```python
from build123d import *

# Parameters (mm, degrees)
SKETCH1_W           = 50
SKETCH1_H           = 10
BOSS_EXTRUDE1_DEPTH = 60
CHAMFER1_SIZE       = 3
CHAMFER1_SIZE2      = 8.242432258
CHAMFER2_SIZE       = 3
CHAMFER2_SIZE2      = 8.242432258


with BuildPart() as part:
    # Sketch1 → Boss-Extrude1 (new body)
    with BuildSketch(Plane(origin=(0, 0, 0), x_dir=(0, 0, -1), z_dir=(1, 0, 0))):
        Rectangle(SKETCH1_W, SKETCH1_H)
    extrude(amount=BOSS_EXTRUDE1_DEPTH)

    # Chamfer1
    chamfer1_edges = [part.edges().sort_by_distance(p)[0] for p in [
        (30, 5, 25),
    ]]
    chamfer1_side = [part.faces().sort_by_distance(p)[0] for p in [
        (30, 5, 0),
    ]]
    chamfer(chamfer1_edges, length=CHAMFER1_SIZE, length2=CHAMFER1_SIZE2, reference=chamfer1_side[0])

    # Chamfer2
    chamfer2_edges = [part.edges().sort_by_distance(p)[0] for p in [
        (30, 5, -25),
    ]]
    chamfer2_side = [part.faces().sort_by_distance(p)[0] for p in [
        (30, 5, -1.5),
    ]]
    chamfer(chamfer2_edges, length=CHAMFER2_SIZE, length2=CHAMFER2_SIZE2, reference=chamfer2_side[0])


solid = part.part
```
Check sheet for the modelled part. Datum: model origin and axes. Units: mm. Round coordinates to 2 decimals unless told otherwise and drop trailing zeros. Loops run counter-clockwise (first coordinate to the right, second up) from the corner with the lowest first, then second, coordinate; pieces in that order, holes last. Notation, with made-up numbers: M 79,83.5 L 108,83.5 A12 cw 108,100.5 Z; hole C 6.5,-20 d10. An arc over 180 degrees is marked long. Answer as a JSON object with one key per item and string values.
1. Gauge pin test, flat ends, axial feed: P1, Ø1, axis at x = 43, y = 2.5, coming from the -Z side; P2, Ø1.5, axis at x = 53, y = -2, coming from the +Z side. Record the tip position at first contact, or that the pin passes through.
Reply:
{"P1": "stops at z = -23.09", "P2": "stops at z = 24.82"}
2. Scan lines: line 1 (Z direction, x = 30.5, y = 2); line 2 (Z direction, x = 50, y = 0.5). Record each from-to range of solid material in increasing order.
Reply:
{"line 1": "z = -23.09 to 23.09", "line 2": "z = -23.64 to 23.64"}
3. Section check A-A (x = 19.5). Record the boundary of the cut face in (y, z).
Reply:
{"outline": "M -5,-25 L -3.24,-25 L 5,-22 L 5,22 L -3.24,25 L -5,25 Z"}
4. Section check C-C (y = 2.5). Record the boundary of the cut face in (x, z).
Reply:
{"outline": "M 0,-22.91 L 60,-22.91 L 60,22.91 L 0,22.91 Z"}
5. Section check B-B (y = -2). Record the boundary of the cut face in (x, z).
Reply:
{"outline": "M 0,-24.55 L 60,-24.55 L 60,24.55 L 0,24.55 Z"}
